Check sheet for the drawn part. Datum: minimum x, y, z corner. Units: mm. A direction names the side the tool comes from. Round coordinates to 2 decimals unless told otherwise and drop trailing zeros. Write each loop counter-clockwise with the first axis right and the second up, starting at its lowest first coordinate (ties: lowest second). Pieces come first, ordered by that corner, then holes. Notation, with made-up numbers: (23, 67) -> (48, 67) arc R19 cw to (48, 88) -> close; hole circle Ø8 at (9.25, 83.5). An arc over 180 degrees is marked (long way). Use a Markdown table: item, result.
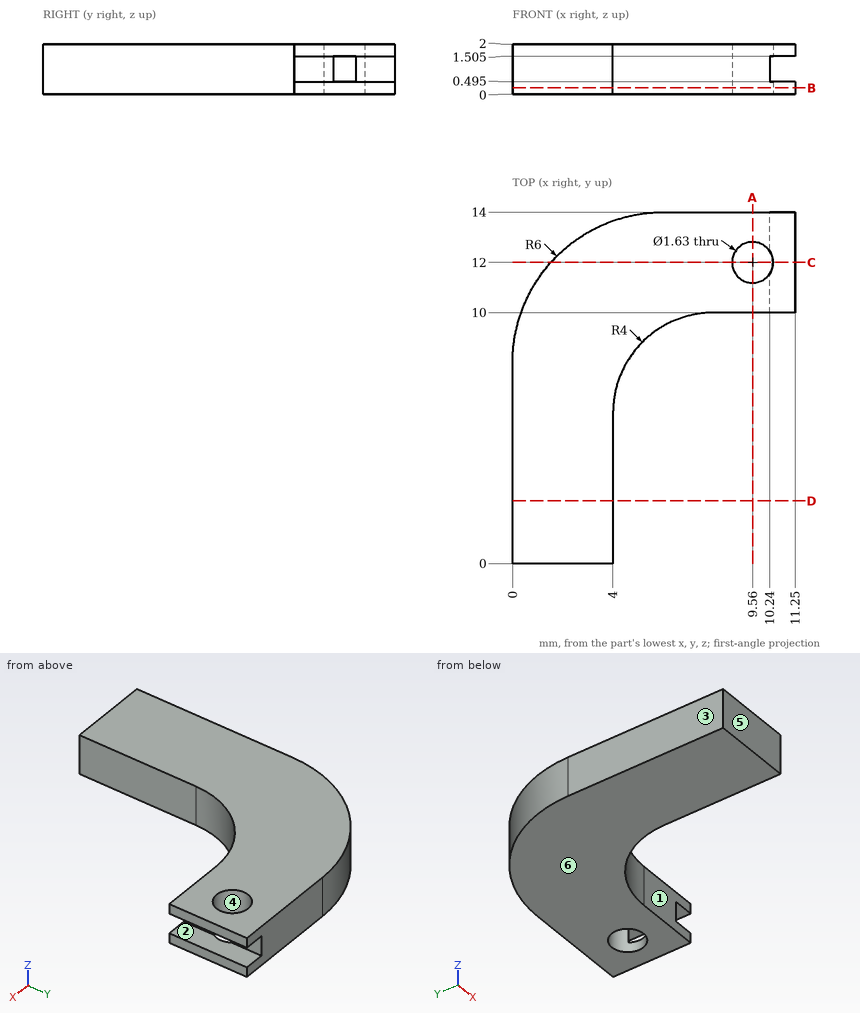
(1) Section check A-A on x = 9.56. Record the cut outline in (y, z) (3 decimals), plus the area to 3 significant figures.
A:
| item | result |
|---|---|
| outline | (10, 0) -> (11.185, 0) -> (11.185, 2) -> (10, 2) -> close; (12.815, 0) -> (14, 0) -> (14, 2) -> (12.815, 2) -> close |
| area | 4.74 mm2 |
(2) Thickness scan on line 1 (Y direction, x = 9.56, z = 0.4) (3 decimals); line 2 (X direction, y = 1, z = 0.8); line 3 (X direction, y = 8.5, z = 1.7). Record the ranges inside material, lowest first.
A:
| item | result |
|---|---|
| line 1 | y = 10 to 11.185, 12.815 to 14 |
| line 2 | x = 0 to 4 |
| line 3 | x = 0.02 to 4.88 |
(3) Release check for a two-part mould opening along Y. For the marked faces 4, 5 and 6 record: +Y half, -Y half, draft (parallel to the pull), parting line (faces both ways), or undercut.
A:
| item | result |
|---|---|
| face 4 | undercut |
| face 5 | -Y half |
| face 6 | draft |
(4) Section check B-B on z = 0.25. Record the cut outline in (x, y) (3 decimals).
A:
| item | result |
|---|---|
| outline | (0, 0) -> (4, 0) -> (4, 6) arc R4 cw to (8, 10) -> (11.25, 10) -> (11.25, 14) -> (6, 14) arc R6 ccw to (0, 8) -> close; hole circle Ø1.63 at (9.56, 12) |
(5) Section check C-C on y = 12. Record the cut outline in (x, z) (3 decimals), plus the area to 3 significant figures.
A:
| item | result |
|---|---|
| outline | (1.528, 0) -> (8.745, 0) -> (8.745, 2) -> (1.528, 2) -> close; (10.375, 0) -> (11.25, 0) -> (11.25, 0.495) -> (10.375, 0.495) -> close; (10.375, 1.505) -> (11.25, 1.505) -> (11.25, 2) -> (10.375, 2) -> close |
| area | 15.3 mm2 |
(6) Access from +Z, -Z, +X, -X, +Y, -Y to the whole of each face (thin tool, end or side, straight path). Record for the marked faces 1, 2 and 3.
A:
| item | result |
|---|---|
| face 1 | +Z, -Z, +X, -Y |
| face 2 | +X, +Y, -Y |
| face 3 | +Z, -Z, -X, +Y, -Y |
(7) Section check D-D on y = 2.5. Record the cut outline in (x, z), plus the area to 3 significant figures.
A:
| item | result |
|---|---|
| outline | (0, 0) -> (4, 0) -> (4, 2) -> (0, 2) -> close |
| area | 8.00 mm2 |
